Input: part model. Units: mm. Frame: model coordinates. Coordinates: 2 decimals unless noted, no trailing zeros. Write each loop counter-clockwise with the first axis right and the second up, starting at its lowest first coordinate (ties: lowest second). Pieces come first, ordered by that corner, then holes.
1) Line query: L1, parallel to Z at x = 1.5, y = -178; L2, parallel to Y at x = 3, z = 377.5. Output: solid intervals per line, ascending.
2) Section query A-A (z = -4). Output: boundary loops of the cut face in (x, y), then the cut area to 3 significant figures.
3) Section query C-C (x = -2.75). Output: boundary loops of the cut face in (y, z), then the cut area to 3 significant figures.
4) Section query B-B (y = -151.5). Output: boundary loops of the cut face in (x, z).
from build123d import *

# Parameters (mm, degrees)
F0_W     = 1397
F0_H     = 977.9
F1_DEPTH = 6.35
F2_W     = 762
F2_H     = 762
F3_DEPTH = 12.701


with BuildPart() as f1:
    # F0 (on Right) → F1 (new body, symmetric)
    with BuildSketch(Plane.YZ):
        Rectangle(F0_W, F0_H)
    extrude(amount=F1_DEPTH, both=True)

    # F2 (on face) → F3 (cut, through all)
    with BuildSketch(Plane.YZ.offset(6.35)):
        with Locations((38.1, 0)):
            Rectangle(F2_W, F2_H)
    extrude(amount=-F3_DEPTH, mode=Mode.SUBTRACT)


solid = f1.part
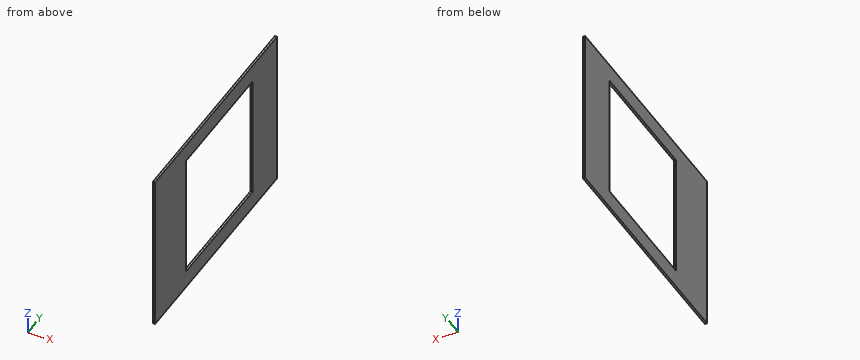
Answer:
1. L1: z = -488.95 to -381, 381 to 488.95
1. L2: y = -698.5 to -342.9, 419.1 to 698.5
2. outline: (-6.35, -698.5) - (6.35, -698.5) - (6.35, -342.9) - (-6.35, -342.9) - close; (-6.35, 419.1) - (6.35, 419.1) - (6.35, 698.5) - (-6.35, 698.5) - close
2. area: 8,060 mm2
3. outline: (-698.5, -488.95) - (698.5, -488.95) - (698.5, 488.95) - (-698.5, 488.95) - close; hole (-342.9, -381) - (419.1, -381) - (419.1, 381) - (-342.9, 381) - close
3. area: 785,000 mm2
4. outline: (-6.35, -488.95) - (6.35, -488.95) - (6.35, -381) - (-6.35, -381) - close; (-6.35, 381) - (6.35, 381) - (6.35, 488.95) - (-6.35, 488.95) - close
